Source: CAD feature listing. Evaluate the final solid. Frame: model axes, mm. A direction names the side the tool comes from. Give positions to 0.01 mm unless a question says otherwise; leave off trailing zeros. Loops run counter-clockwise (first coordinate to the right, second up) from the corner with the lowest first, then second, coordinate; pieces in that order, holes last. Notation, with made-up numbers: M 33,7 L 48,7 A31 ccw 48,40 Z; hole C 81.5,-15.5 d1. An arc over 180 degrees is marked long. Answer in a Markdown table with one row per item.
```python
from build123d import *

# Parameters (mm, degrees)
F1_DEPTH  = 100
F2_W      = 110
F2_H      = 110
F3_DEPTH  = 4
F4_W      = 17
F4_H      = 4.05
F5_DEPTH  = 4
F7_D      = 4
F8_R      = 7.5
F9_DEPTH  = 25
F11_D     = 2.5
F11_DEPTH = 12
F11_TIP   = 0.7510757738


with BuildPart() as f1:
    # F0 (on Top) → F1 (new body)
    with BuildSketch(Plane.XY):
        Polygon((0, 48.925), (0, 0), (110, 0), (110, 50.5), (114, 46.5), (114, 63.5), (110, 59.5), (110, 110), (0, 110), (0, 61.075), (5, 64.075), (5, 45.925), align=None)
        with BuildLine():
            ThreePointArc((4, 101), (5.4644660941, 104.5355339059), (9, 106))
            Line((9, 106), (101, 106))
            ThreePointArc((101, 106), (104.5355339059, 104.5355339059), (106, 101))
            Line((106, 101), (106, 9))
            ThreePointArc((106, 9), (104.5355339059, 5.4644660941), (101, 4))
            Line((101, 4), (9, 4))
            ThreePointArc((9, 4), (5.4644660941, 5.4644660941), (4, 9))
            Line((4, 9), (4, 40))
            Line((4, 40), (6, 40))
            ThreePointArc((6, 40), (6.7071067812, 40.2928932188), (7, 41))
            Line((7, 41), (7, 69))
            ThreePointArc((7, 69), (6.7071067812, 69.7071067812), (6, 70))
            Line((6, 70), (4, 70))
            Line((4, 70), (4, 101))
        make_face(mode=Mode.SUBTRACT)
    extrude(amount=F1_DEPTH)

    # F2 (on Top) → F3 (join)
    with BuildSketch(Plane.XY):
        with Locations((55, 55)):
            Rectangle(F2_W, F2_H)
    extrude(amount=F3_DEPTH)

    # F4 (on face) → F5 (cut)
    with BuildSketch(Plane.YZ.offset(114)):
        with Locations((55, 2.025)):
            Rectangle(F4_W, F4_H)
    extrude(amount=-F5_DEPTH, mode=Mode.SUBTRACT)

    # F7 (through all)
    with Locations(Plane.YZ.offset(114)):
        with Locations((54.5, 92)):
            Hole(F7_D / 2)

    # F8 (on face) → F9 (cut)
    with BuildSketch(Plane.XZ):
        with Locations((55, 14)):
            Circle(F8_R)
    extrude(amount=-F9_DEPTH, mode=Mode.SUBTRACT)

    # F11
    with Locations(Plane.XY.offset(100)):
        with Locations((4, 106), (106, 106), (106, 4), (4, 4)):
            Hole(F11_D / 2, depth=F11_DEPTH)
            with Locations((0, 0, -(F11_DEPTH + F11_TIP / 2))):  # 118° drill point
                Cone(0, F11_D / 2, F11_TIP, mode=Mode.SUBTRACT)


solid = f1.part
```
Q1. Contact query for flat-ended pins moving along their axis: pin 1 Ø1.2 at (x, y) = (112.5, 56) entering from -Z; pin 2 Ø2 at (x, y) = (95, 12) entering from +Z; pin 3 Ø2 at (y, z) = (65, 89.5) entering from +X. Output: stop coordinate, or through.
Values follow:
| item | result |
|---|---|
| pin 1 | z = 4.05 |
| pin 2 | z = 4 |
| pin 3 | x = 110 |
Q2. Mould query, pull axis Z, two halves, no side actions, for faces 4 (the flat face through (54, 56, 4)), 5 (the cylindrical face through (109.944, 54.76, 93.983)), 6 (the flat face through (0, 68, 49)). Classes: +Z half, -Z half, draft (parallel to the pull), parting line (faces both ways), or undercut.
Values follow:
| item | result |
|---|---|
| face 4 | +Z half |
| face 5 | undercut |
| face 6 | draft |
Q3. Section query A-A (x = 55). Output: boundary loops of the cut face in (y, z), plus the area to 3 significant figures.
Values follow:
| item | result |
|---|---|
| outline | M 0,0 L 110,0 L 110,100 L 106,100 L 106,4 L 4,4 L 4,6.5 L 0,6.5 Z; M 0,21.5 L 4,21.5 L 4,100 L 0,100 Z |
| area | 1,150 mm^2 |
Q4. Ray query, probe 1 along X at (y, z) = (38.5, 50); probe 2 along X at (y, z) = (54.5, 16.5). Return the intervals inside material, ascending. Write a range as from..to.
Values follow:
| item | result |
|---|---|
| probe 1 | 0..4, 106..110 |
| probe 2 | 5..7, 106..114 |
Q5. Section query D-D (z = 28.5). Output: boundary loops of the cut face in (x, y) (3 decimals).
Values follow:
| item | result |
|---|---|
| outline | M 0,0 L 110,0 L 110,50.5 L 114,46.5 L 114,63.5 L 110,59.5 L 110,110 L 0,110 L 0,61.075 L 5,64.075 L 5,45.925 L 0,48.925 Z; hole M 4,9 A5 ccw 9,4 L 101,4 A5 ccw 106,9 L 106,101 A5 ccw 101,106 L 9,106 A5 ccw 4,101 L 4,70 L 6,70 A1 cw 7,69 L 7,41 A1 cw 6,40 L 4,40 Z |
Q6. Reachability of faces 1 (the cylindrical face through (53.37, 1.97, 6.68)), 2 (the flat face through (7, 55, 51)), 3 (the flat face through (112, 55, 4.05)) from +Z, -Z, +X, -X, +Y, -Y: full face, straight path, thin tool, end or side. Return the list, or none.
Values follow:
| item | result |
|---|---|
| face 1 | -Y |
| face 2 | +Z |
| face 3 | -Z, +X, +Y, -Y |
Q7. Section query B-B (y = 54.5). Output: boundary loops of the cut face in (x, z).
Values follow:
| item | result |
|---|---|
| outline | M 0,0 L 110,0 L 110,4.05 L 114,4.05 L 114,90 L 106,90 L 106,4 L 7,4 L 7,90 L 5,90 L 5,4 L 0,4 Z; M 5,94 L 7,94 L 7,100 L 5,100 Z; M 106,94 L 114,94 L 114,100 L 106,100 Z |
